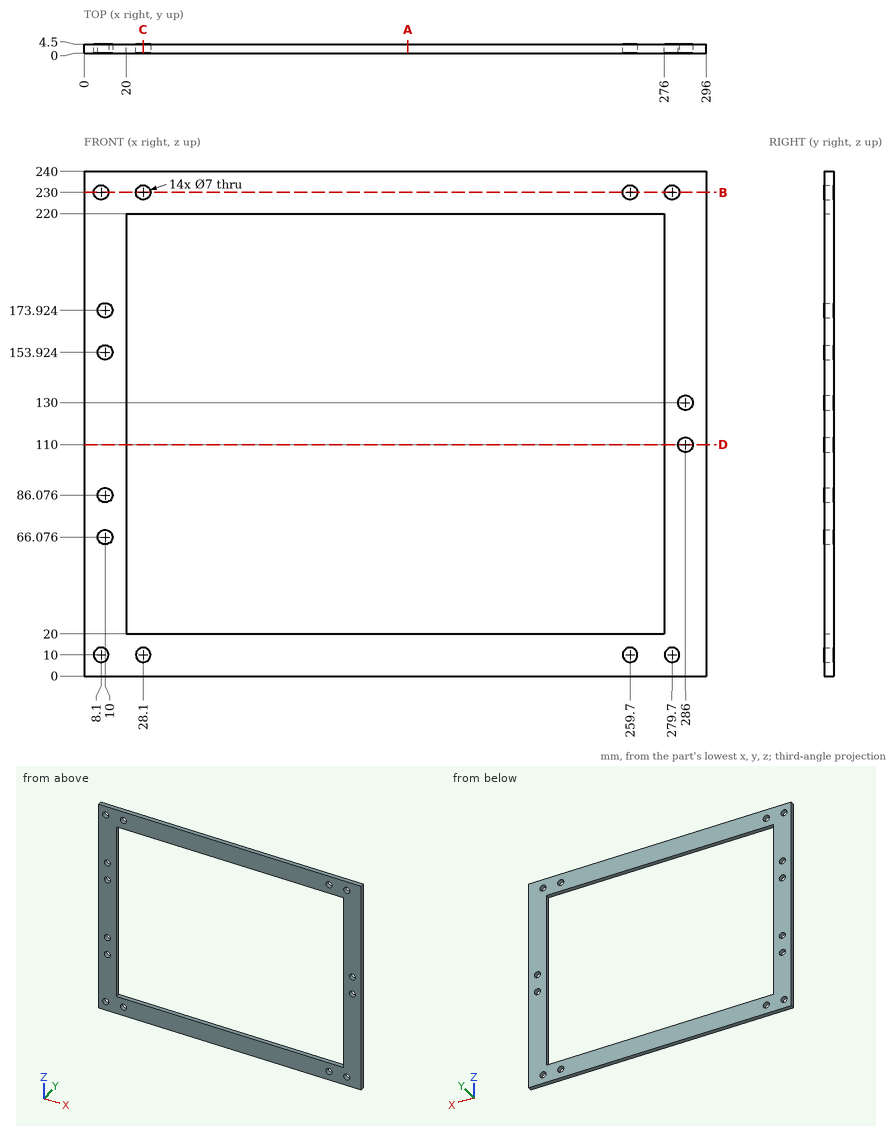
Design review of the part shown in the three views and the two pictorial views. Dimensions are in mm from the part's minimum x, y and z. Round coordinates to 2 decimals unless told otherwise and drop trailing zeros. Write each loop counter-clockwise with the first axis right and the second up, starting at its lowest first coordinate (ties: lowest second). Pieces come first, ordered by that corner, then holes. Notation, with made-up numbers: (-11.5, 35.25) -> (40.5, 35.25) arc R14 ccw to (40.5, 43.25) -> close; hole circle Ø7 at (77.25, -18.75). An arc over 180 degrees is marked (long way). Write item = value, one per line. Start each with the question number.
1) Clearance check with flat-ended pins moving along their axes: pin 1 (1.3 mm diameter, centred on x = 208.5, y = 3, fed in from -Z); pin 2 (4 mm diameter, centred on x = 10, z = 86.08, fed in from -Y). State where each tip first meets the part, or that it passes through.
2) Take a section at D-D, the plane z = 110. State the section outline as (x, y) points, plus the area to 4 significant figures.
3) Take a section at A-A, the plane x = 154. State the section outline as (y, z) points, plus the area to 3 significant figures.
4) Take a section at B-B, the plane z = 230. State the section outline as (x, y) points.
5) Wall thickness on probe 1 along X at (y, z) = (3.55, 174); probe 2 along Z at (x, y) = (279.7, 1.95); probe 3 along Z at (x, y) = (259.7, 1.65): over which ranges is each line inside the solid? List them lowest first. Write a range as from..to.
6) Take a section at C-C, the plane x = 28.1. State the section outline as (y, z) points.
Results list:
q1.pin_1 = 0
q1.pin_2 = through
q2.outline = (0, 0) -> (20, 0) -> (20, 4.5) -> (0, 4.5) -> close; (276, 0) -> (282.5, 0) -> (282.5, 4.5) -> (276, 4.5) -> close; (289.5, 0) -> (296, 0) -> (296, 4.5) -> (289.5, 4.5) -> close
q2.area = 148.5 mm²
q3.outline = (0, 0) -> (4.5, 0) -> (4.5, 20) -> (0, 20) -> close; (0, 220) -> (4.5, 220) -> (4.5, 240) -> (0, 240) -> close
q3.area = 180 mm²
q4.outline = (0, 0) -> (4.6, 0) -> (4.6, 4.5) -> (0, 4.5) -> close; (11.6, 0) -> (24.6, 0) -> (24.6, 4.5) -> (11.6, 4.5) -> close; (31.6, 0) -> (256.2, 0) -> (256.2, 4.5) -> (31.6, 4.5) -> close; (263.2, 0) -> (276.2, 0) -> (276.2, 4.5) -> (263.2, 4.5) -> close; (283.2, 0) -> (296, 0) -> (296, 4.5) -> (283.2, 4.5) -> close
q5.probe_1 = 0..6.5, 13.5..20, 276..296
q5.probe_2 = 0..6.5, 13.5..226.5, 233.5..240
q5.probe_3 = 0..6.5, 13.5..20, 220..226.5, 233.5..240
q6.outline = (0, 0) -> (4.5, 0) -> (4.5, 6.5) -> (0, 6.5) -> close; (0, 13.5) -> (4.5, 13.5) -> (4.5, 20) -> (0, 20) -> close; (0, 220) -> (4.5, 220) -> (4.5, 226.5) -> (0, 226.5) -> close; (0, 233.5) -> (4.5, 233.5) -> (4.5, 240) -> (0, 240) -> close
